from build123d import *

# Parameters (mm, degrees)
F2_W     = 4.05
F2_H     = 8.1
F3_DEPTH = 6
F4_R     = 0.75
F5_R     = 0.5


with BuildPart() as f1:
    # F0 (on Front) → F1 (revolve)
    with BuildSketch(Plane.XZ):
        Polygon((4.05, 0), (4.05, 6), (5.5, 7), (10.5, 7), (9.056624327, 9.5), (0, 9.5), (0, 0), align=None)
    revolve(axis=Axis((0, 0, 4.75), (0, 0, -1)))

    # F2 (on face) → F3 (cut)
    with BuildSketch(Plane(origin=(0, 0, 0), x_dir=(1, 0, 0), z_dir=(0, 0, -1))):
        with Locations((2.025, 0)):
            Rectangle(F2_W, F2_H)
    extrude(amount=-F3_DEPTH, mode=Mode.SUBTRACT)

    # F4
    f4_edges = [f1.edges().sort_by_distance(p)[0] for p in [
        (0, 0, 0),
        (0, 0, 6),
        (-4.05, 0, 0),
    ]]
    fillet(f4_edges, radius=F4_R)

    # F5
    f5_edges = [f1.edges().sort_by_distance(p)[0] for p in [
        (-9.056624, 0, 9.5),
        (-10.5, 0, 7),
    ]]
    fillet(f5_edges, radius=F5_R)


solid = f1.part
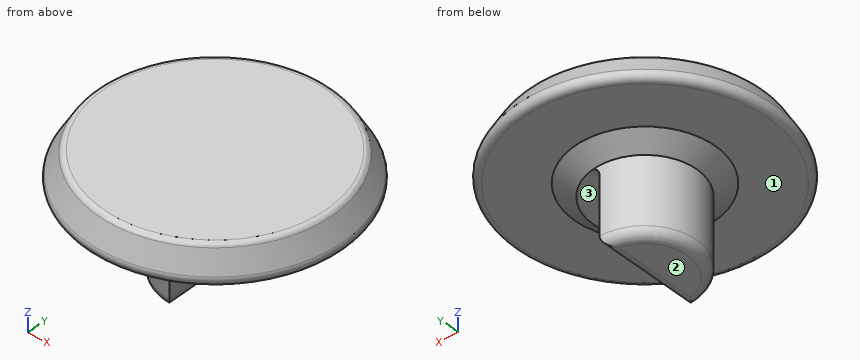
Check sheet for the modelled part. Datum: model origin and axes. Units: mm. Face numbers are marked on the shaded views. A direction names the side the tool comes from. Coordinates: 2 decimals unless noted, no trailing zeros. Loops run counter-clockwise (first coordinate to the right, second up) from the corner with the lowest first, then second, coordinate; pieces in that order, holes last. Notation, with made-up numbers: (-18, 29) -> (10, 29) arc R11 ccw to (10, 35) -> close; hole circle Ø10 at (41, 31). An arc over 180 degrees is marked (long way). Write item = value, one per line. Start each with the question number.
1. Section check B-B on z = 5. Record the cut outline in (x, y), then the cut area to 3 significant figures.
2. Section check A-A on y = 0. Record the cut outline in (x, z), then the cut area to 3 significant figures.
3. Tool access check on the marked faces 1, 2 and 3. Record the directions out of +Z, -Z, +X, -X, +Y, -Y that give a thin tool (end or side, any length) a straight path to the whole face; none if there is none.
4. Material ranges on line 1 (Z direction, x = 2.25, y = -0.5); line 2 (Z direction, x = 7.5, y = 4.5); line 3 (Y direction, x = -6.5, z = 7.5), recorded low to high.
5. Depth check by flat-ended pin: P1, Ø1.6, axis at x = 1.5, y = 0, coming from the -Z side; P2, Ø1.5, axis at x = -1, z = 7.5, coming from the +Y side; P3, Ø3.5, axis at y = 1.5, z = 3.5, coming from the +X side. Enter the tip coordinate at first touch or a pass-through.
6. Section check C-C on z = 7.5. Record the cut outline in (x, y), then the cut area to 3 significant figures.
Responses:
q1.outline = (0, -4.05) -> (0, 4.05) arc R4.05 ccw to start
q1.area = 25.8 mm2
q2.outline = (-10.07, 7.75) arc R0.5 ccw to (-9.63, 7) -> (-5.5, 7) -> (-4.05, 6) -> (-4.05, 0.75) arc R0.75 ccw to (-3.3, 0) -> (-0.75, 0) arc R0.75 ccw to (0, 0.75) -> (0, 5.25) arc R0.75 cw to (0.75, 6) -> (4.05, 6) -> (5.5, 7) -> (9.63, 7) arc R0.5 ccw to (10.07, 7.75) -> (9.2, 9.25) arc R0.5 ccw to (8.77, 9.5) -> (-8.77, 9.5) arc R0.5 ccw to (-9.2, 9.25) -> close
q2.area = 82.3 mm2
q3.face_1 = -Z
q3.face_2 = -Z, +X, -X, +Y, -Y
q3.face_3 = -Z, +X, +Y, -Y
q4.line_1 = 6 to 9.5
q4.line_2 = 7 to 9.5
q4.line_3 = -7.77 to 7.77
q5.P1 = 6
q5.P2 = 10.13
q5.P3 = 0
q6.outline = circle Ø20.27 at (0, 0)
q6.area = 323 mm2
